Work out the finished part from the listing and answer in its coordinate system (mm). A direction names the side the tool comes from. Give positions to 0.01 mm unless a question says otherwise; leave off trailing zeros. Write each loop counter-clockwise with the first axis right and the second up, starting at its lowest first coordinate (ties: lowest second). Pieces come first, ordered by that corner, then holes.
1) Find section C-C (z = 1.5). Count the separate pieces of the cut face and the enclosed holes in it, plus the area to 3 significant figures.
2) Determine the mould class of faces 3 (the face through (-29.97, -1.32, 2.46)), 4 (the face through (3, 6, 1)), 5 (the face through (6, -6, 0)), 6 (the face through (-10, -3.2, 3.8)) for opening direction Y: pulls with the +Y half, pulls with the -Y half, needs draft (parallel to the pull), parting line crosses it, or undercut.
3) Given pin 1 Ø1 at (y, z) = (17, 1.5) entering from -X; pin 2 Ø3 at (x, y) = (-3, -7) entering from +Z; pin 3 Ø1.5 at (x, z) = (-6, 3) entering from +Y, each flat-ended and moving along its own axis, determine where each tip first touches the part or whether it passes through.
4) Straight lines are drawn through the part: probe 1 along Y at (x, z) = (7, 1.6); probe 2 along Z at (x, y) = (5, -1.5); probe 3 along Y at (x, z) = (6.5, 0.65). For each, find the intervals that lie inside material, in ascending order.
5) Find section A-A (x = 0). Determine the outline of the cut face in (y, z).
6) Find section D-D (y = 26). Determine the outline of the cut face in (x, z), plus the area to 3 significant figures.
7) A tool of negligible diameter and unlimited length cuts with its end or side. For faces 1 (the face through (3, -8, 1)), 2 (the face through (-5, 0, 2.5)), from which of +Z, -Z, +X, -X, +Y, -Y can it reach the whole face along a straight path? Write none if from no direction.
Autodesk Fusion 360 part; units mm, degrees
sketch "Sketch1" plane through (0, 0, 0) normal (0, 0, 1) x (1, 0, 0)
  circle A0 centre (0, 0) radius 30
  circle A1 centre (0, 0) radius 4.5
  line L0 (7, -7) -> (-7, -7)
  line L1 (-7, -7) -> (-7, 7)
  line L2 (-7, 7) -> (7, 7)
  line L3 (7, 7) -> (7, -7)
  line L4 (7, -7) -> (-7, 7) construction
  line L5 (-7, -7) -> (7, 7) construction
  line L6 (7, 0) -> (7, 4)
  line L7 (7, 0) -> (7, -4)
  circle A2 centre (7, 3) radius 1
  circle A3 centre (7, 0) radius 1
  circle A4 centre (7, -3) radius 1
  circle A5 centre (-3, 7) radius 1
  circle A6 centre (0, 7) radius 1
  circle A7 centre (3, 7) radius 1
  circle A8 centre (-7, -3) radius 1
  circle A9 centre (-7, 0) radius 1
  circle A10 centre (-7, 3) radius 1
  circle A11 centre (3, -7) radius 1
  circle A12 centre (0, -7) radius 1
  circle A13 centre (-3, -7) radius 1
  dimension "d1" = 60
  dimension "d2" = 9
  dimension "d3" = 14
  dimension "d4" = 14
  dimension "d5" = 4
  dimension "d6" = 4
  dimension "d7" = 2
  dimension "d8" = 2
  dimension "d11" = 0
  dimension "d12" = 0
  dimension "d14" = 360
extrude "Extrude1" add sketch "Sketch1" along normal blind 5 contours A0 | L0 L1 L2 L3 L6 L7 A2 A3 A4 A5 A6 A7 A8 A9 A10 A11 A12 A13
sketch "Sketch2" plane through (0, 0, 5) normal (0, 0, 1) x (-1, 0, 0)
  circle A0 centre (-7, 3) radius 1
  circle A1 centre (3, 7) radius 1
  circle A2 centre (0, 7) radius 1
  circle A3 centre (0, -7) radius 1
  circle A4 centre (-3, 7) radius 1
  circle A5 centre (3, -7) radius 1
  circle A6 centre (0, 0) radius 4.5
  circle A7 centre (-7, -3) radius 1
  circle A8 centre (-7, 0) radius 1
  circle A9 centre (7, 0) radius 1
  circle A10 centre (-3, -7) radius 1
  circle A11 centre (7, -3) radius 1
  circle A12 centre (7, 3) radius 1
  circle A13 centre (0, 0) radius 30
  circle A14 centre (0, 0) radius 10.5
  dimension "d17" = 21
extrude "Extrude2" cut sketch "Sketch2" against normal blind 2.5 contours A14
Results:
1. separate pieces: 1
1. enclosed holes: 13
1. area: 2,730 mm2
2. face 3: parting line crosses it
2. face 4: undercut
2. face 5: needs draft
2. face 6: undercut
3. pin 1: stops at x = -25.05
3. pin 2: stops at z = 2.5
3. pin 3: stops at y = 29.54
4. probe 1: y = -29.17 to -4, -2 to -1, 1 to 2, 4 to 29.17
4. probe 2: z = 0 to 2.5
4. probe 3: y = -29.29 to -3.87, -2.13 to -0.87, 0.87 to 2.13, 3.87 to 29.29
5. outline: (-30, 0) - (-8, 0) - (-8, 2.5) - (-10.5, 2.5) - (-10.5, 5) - (-30, 5) - close; (-6, 0) - (-4.5, 0) - (-4.5, 2.5) - (-6, 2.5) - close; (4.5, 0) - (6, 0) - (6, 2.5) - (4.5, 2.5) - close; (8, 0) - (30, 0) - (30, 5) - (10.5, 5) - (10.5, 2.5) - (8, 2.5) - close
6. outline: (-14.97, 0) - (14.97, 0) - (14.97, 5) - (-14.97, 5) - close
6. area: 150 mm2
7. face 1: +Z, -Z
7. face 2: +Z
